For this review, use the dimensioned drawing (mm, ordinates from the lowest corner) and the shaded views. Round coordinates to 2 decimals unless told otherwise and drop trailing zeros. Write each loop counter-clockwise with the first axis right and the second up, starting at its lowest first coordinate (ties: lowest second). Pieces come first, ordered by that corner, then holes. Notation, with made-up numbers: (-18, -17.75) -> (-5, -17.75) arc R28 ccw to (-5, 20.25) -> close; hole circle Ø7 at (-11.75, 86). An arc over 180 degrees is marked (long way). Write each question's results on one line, items separated by ' | '. Start each with the question number.
Item 1: Add section B-B (z = 40.28). State the section outline as (x, y) points.
Item 2: To check wall thickness, follow line 1 along X through (y, z) = (2.5, 40.28); line 2 along Z through (x, y) = (37.5, 2.6); line 3 along X through (y, z) = (1.55, 35). State the ranges of each line that lie inside material, in increasing order.
Item 3: Clearance check with flat-ended pins moving along their axes: pin 1 (1 mm diameter, centred on y = 1.5, z = 59, fed in from -X); pin 2 (2 mm diameter, centred on y = 3, z = 59, fed in from -X). State where each tip first meets the part, or that it passes through.
Item 4: Add section A-A (x = 40.28). State the section outline as (y, z) points, plus the area to 3 significant figures.
Item 5: Add section C-C (y = 2.65). State the section outline as (x, z) points, plus the area to 3 significant figures.
Item 6: Add section D-D (z = 49.5). State the section outline as (x, y) points, plus the area to 3 significant figures.
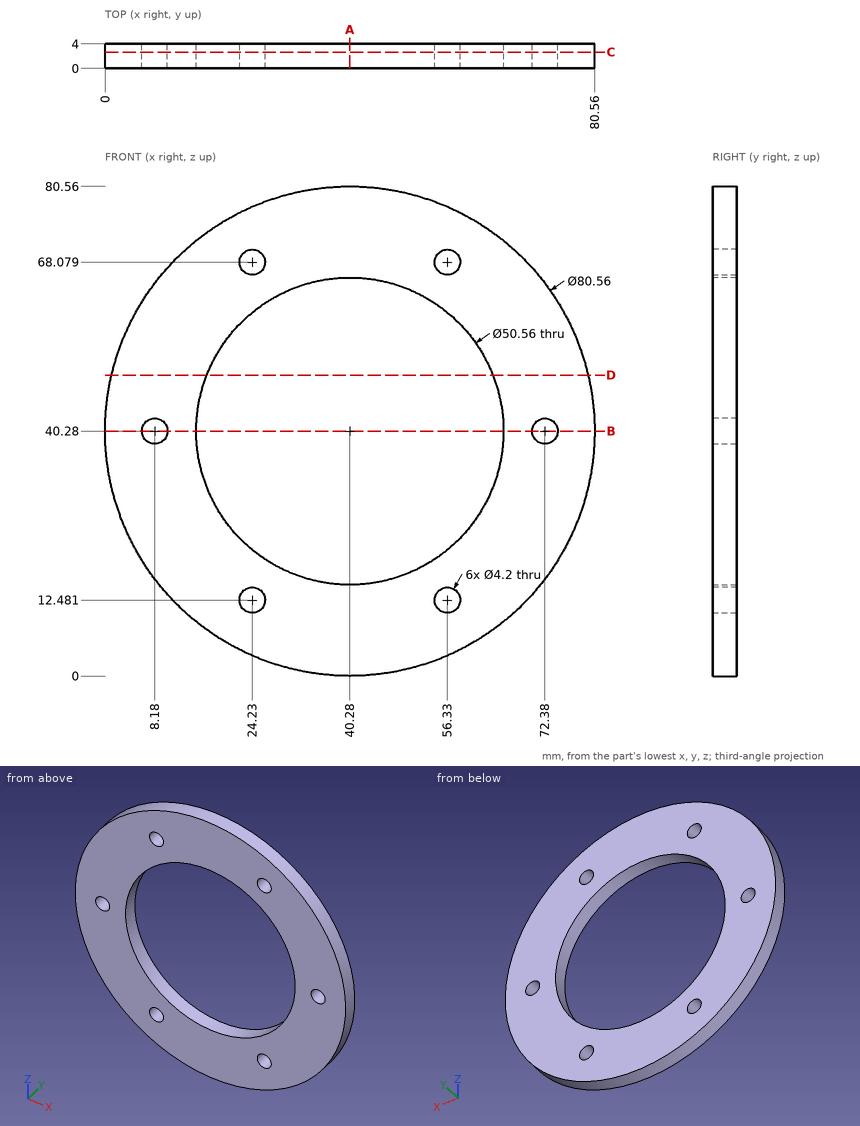
Responses:
1) outline: (0, 0) -> (6.08, 0) -> (6.08, 4) -> (0, 4) -> close; (10.28, 0) -> (15, 0) -> (15, 4) -> (10.28, 4) -> close; (65.56, 0) -> (70.28, 0) -> (70.28, 4) -> (65.56, 4) -> close; (74.48, 0) -> (80.56, 0) -> (80.56, 4) -> (74.48, 4) -> close
2) line 1: x = 0 to 6.08, 10.28 to 15, 65.56 to 70.28, 74.48 to 80.56 | line 2: z = 0.1 to 15.15, 65.41 to 80.46 | line 3: x = 0.35 to 15.56, 65 to 80.21
3) pin 1: stops at x = 4.36 | pin 2: stops at x = 4.11
4) outline: (0, 0) -> (4, 0) -> (4, 15) -> (0, 15) -> close; (0, 65.56) -> (4, 65.56) -> (4, 80.56) -> (0, 80.56) -> close | area: 120 mm^2
5) outline: circle Ø80.56 at (40.28, 40.28); hole circle Ø4.2 at (8.18, 40.28); hole circle Ø50.56 at (40.28, 40.28); hole circle Ø4.2 at (24.23, 12.48); hole circle Ø4.2 at (24.23, 68.08); hole circle Ø4.2 at (56.33, 12.48); hole circle Ø4.2 at (56.33, 68.08); hole circle Ø4.2 at (72.38, 40.28) | area: 3,010 mm^2
6) outline: (1.07, 0) -> (16.74, 0) -> (16.74, 4) -> (1.07, 4) -> close; (63.82, 0) -> (79.49, 0) -> (79.49, 4) -> (63.82, 4) -> close | area: 125 mm^2
